```python
from build123d import *

# Parameters (mm, degrees)
BOSS_EXTRUDE1_DEPTH            = 17
BOSS_EXTRUDE2_START            = 17
SKETCH1_3_W                    = 18
SKETCH1_3_H                    = 7.7
BOSS_EXTRUDE2_DEPTH            = 8
SKETCH9_W                      = 65
SKETCH9_H                      = 70
CUT_EXTRUDE5_DEPTH             = 2
CBORE_FOR_M3_SHCS2_D           = 3.4
CBORE_FOR_M3_SHCS2_CBORE_D     = 6.5
CBORE_FOR_M3_SHCS2_CBORE_DEPTH = 3
SKETCH4_R                      = 1
CUT_EXTRUDE3_DEPTH             = 0.7
CUT_EXTRUDE4_DEPTH             = 0.5
CUT_EXTRUDE4_DEPTH_BACK        = 1
SKETCH6_W                      = 23.342383579
SKETCH6_H                      = 4
CBORE_FOR_M2_SHCS1_D           = 2.4
CBORE_FOR_M2_SHCS1_CBORE_D     = 4.4
CBORE_FOR_M2_SHCS1_CBORE_DEPTH = 2
FILLET1_R                      = 4


with BuildPart() as part:
    # Sketch1 → Boss-Extrude1 (new body)
    with BuildSketch(Plane(origin=(0, 0, 0), x_dir=(1, 0, 0), z_dir=(0, 1, 0))):
        Polygon((32.5, 0.5), (32.5, 70), (15, 90), (-15, 90), (-32.5, 70), (-32.5, -7.7), (-14.5, -7.7), (-14.5, 0), (14.1, 0), (14.1, 0.5), align=None)
    extrude(amount=BOSS_EXTRUDE1_DEPTH)

    # Sketch1<3> → Boss-Extrude2 (add)
    with BuildSketch(Plane(origin=(0, 0, 0), x_dir=(1, 0, 0), z_dir=(0, 1, 0)).offset(BOSS_EXTRUDE2_START)):
        with Locations((-23.5, -3.85)):
            Rectangle(SKETCH1_3_W, SKETCH1_3_H)
    extrude(amount=BOSS_EXTRUDE2_DEPTH)

    # Sketch9 → Cut-Extrude5 (cut)
    with BuildSketch(Plane(origin=(0, 17, 0), x_dir=(1, 0, 0), z_dir=(0, 1, 0))):
        with Locations((0, 35)):
            Rectangle(SKETCH9_W, SKETCH9_H)
    extrude(amount=-CUT_EXTRUDE5_DEPTH, mode=Mode.SUBTRACT)

    # CBORE for M3 SHCS2 (through all)
    with Locations(Plane(origin=(0, 15, 0), x_dir=(1, 0, 0), z_dir=(0, 1, 0))):
        with Locations((-5.12, 20), (12.88, 20), (-5.12, 63.6), (12.88, 63.6), (12.88, 5), (12.88, 48.6)):
            CounterBoreHole(CBORE_FOR_M3_SHCS2_D / 2, CBORE_FOR_M3_SHCS2_CBORE_D / 2, CBORE_FOR_M3_SHCS2_CBORE_DEPTH)

    # Sketch4 → Cut-Extrude3 (cut)
    with BuildSketch(Plane(origin=(0, 0, 0), x_dir=(0, 0, -1), z_dir=(1, 0, 0))):
        with BuildLine():
            ThreePointArc((78.521450009, 2.853281834), (77.510842566, 2.872195508), (77, 2))
            Line((77, 2), (78, 2))
            Line((78, 2), (78.521450009, 2.853281834))
        make_face()
        with BuildLine():
            Line((78, 2), (77, 2))
            ThreePointArc((77, 2), (78, 1), (79, 2))
            ThreePointArc((79, 2), (78.872195508, 2.489157434), (78.521450009, 2.853281834))
            Line((78.521450009, 2.853281834), (78, 2))
        make_face()
        with BuildLine():
            Line((58.012399764, 2.853281834), (57.490949754, 2))
            Line((57.490949754, 2), (58.490949754, 2))
            ThreePointArc((58.490949754, 2), (58.363145263, 2.489157434), (58.012399764, 2.853281834))
        make_face()
        with BuildLine():
            Line((58.490949754, 2), (57.490949754, 2))
            Line((57.490949754, 2), (58.012399764, 2.853281834))
            ThreePointArc((58.012399764, 2.853281834), (56.618754246, 1.510842566), (58.490949754, 2))
        make_face()
        with Locations((57.490949754, 2)):
            Circle(SKETCH4_R)
        with Locations((78, 2)):
            Circle(SKETCH4_R)
        Polygon((57.490949754, 2), (78, 2), (89, 20), (68.490949754, 20), align=None)
    extrude(amount=-CUT_EXTRUDE3_DEPTH, mode=Mode.SUBTRACT)

    # Sketch6 → Cut-Extrude4 (cut, two sides: drawn at the far end of the back side and taken through both)
    with BuildSketch(Plane.ZY.offset(-CUT_EXTRUDE4_DEPTH_BACK)):
        with Locations((-77.828808211, 15)):
            Rectangle(SKETCH6_W, SKETCH6_H)
    extrude(amount=CUT_EXTRUDE4_DEPTH + CUT_EXTRUDE4_DEPTH_BACK, mode=Mode.SUBTRACT)

    # CBORE for M2 SHCS1 (through all)
    with Locations(Plane(origin=(0, 0, 0), x_dir=(-1, 0, 0), z_dir=(0, 0, -1))):
        with Locations((22.5, 20.24)):
            CounterBoreHole(CBORE_FOR_M2_SHCS1_D / 2, CBORE_FOR_M2_SHCS1_CBORE_D / 2, CBORE_FOR_M2_SHCS1_CBORE_DEPTH)

    # Fillet1
    fillet1_edges = [part.edges().sort_by_distance(p)[0] for p in [
        (-32.5, 25, 3.85),
        (-14.5, 25, 3.85),
    ]]
    fillet(fillet1_edges, radius=FILLET1_R)


solid = part.part
```
Model file for the job. Use its own axes, mm. A direction names the side the tool comes from. Coordinates: 2 decimals unless noted, no trailing zeros. Loops run counter-clockwise (first coordinate to the right, second up) from the corner with the lowest first, then second, coordinate; pieces in that order, holes last. Notation, with made-up numbers: (54, 84.5) -> (69, 84.5) arc R27 ccw to (69, 101.5) -> close; hole circle Ø9 at (84, 6). An arc over 180 degrees is marked (long way). Answer as a JSON object with one key per item and string values.
Q1. Cut at D-D (y = 8.5). List the corners of the cut face in (x, z).
Report:
{"outline": "(-32.5, -70) -> (-15, -90) -> (15, -90) -> (32.5, -70) -> (32.5, -0.5) -> (14.1, -0.5) -> (14.1, 0) -> (-14.5, 0) -> (-14.5, 7.7) -> (-32.5, 7.7) -> close; hole circle Ø3.4 at (-5.12, -63.6); hole circle Ø3.4 at (-5.12, -20); hole (-0.7, -81.97) -> (0, -81.97) -> (0, -61.46) -> (-0.7, -61.46) -> close; hole circle Ø3.4 at (12.88, -63.6); hole circle Ø3.4 at (12.88, -48.6); hole circle Ø3.4 at (12.88, -20); hole circle Ø3.4 at (12.88, -5)"}
Q2. Cut at B-B (x = -5.12). List the corners of the cut face in (y, z).
Report:
{"outline": "(0, -90) -> (17, -90) -> (17, -70) -> (15, -70) -> (15, -66.85) -> (12, -66.85) -> (12, -65.3) -> (0, -65.3) -> close; (0, -61.9) -> (12, -61.9) -> (12, -60.35) -> (15, -60.35) -> (15, -23.25) -> (12, -23.25) -> (12, -21.7) -> (0, -21.7) -> close; (0, -18.3) -> (12, -18.3) -> (12, -16.75) -> (15, -16.75) -> (15, 0) -> (0, 0) -> close"}
Q3. Probe probe 1 along Z at (x, y) = (12.88, 8); probe 2 along Z at (x, y) = (12.88, 14.3); probe 3 along X at (y, z) = (13.5, -18.5). List the from-to ranges inside material, lowest first.
Report:
{"probe 1": "z = -90 to -65.3, -61.9 to -50.3, -46.9 to -21.7, -18.3 to -6.7, -3.3 to 0", "probe 2": "z = -90 to -66.85, -60.35 to -51.85, -45.35 to -23.25, -16.75 to -8.25, -1.75 to 0", "probe 3": "x = -32.5 to -8, -2.24 to 10, 15.76 to 32.5"}
Q4. Cut at A-A (z = -48.6). List the corners of the cut face in (x, y), and give its area (3 significant figures).
Report:
{"outline": "(-32.5, 0) -> (11.18, 0) -> (11.18, 12) -> (9.63, 12) -> (9.63, 15) -> (-32.5, 15) -> close; (14.58, 0) -> (32.5, 0) -> (32.5, 15) -> (16.13, 15) -> (16.13, 12) -> (14.58, 12) -> close", "area": "915 mm2"}
Q5. Cut at C-C (z = -63.6). List the corners of the cut face in (x, y), and give its area (3 significant figures).
Report:
{"outline": "(-32.5, 0) -> (-6.82, 0) -> (-6.82, 12) -> (-8.37, 12) -> (-8.37, 15) -> (-32.5, 15) -> close; (-3.42, 0) -> (11.18, 0) -> (11.18, 12) -> (9.63, 12) -> (9.63, 15) -> (-1.87, 15) -> (-1.87, 12) -> (-3.42, 12) -> close; (14.58, 0) -> (32.5, 0) -> (32.5, 15) -> (16.13, 15) -> (16.13, 12) -> (14.58, 12) -> close; hole (-0.7, 2) -> (0, 2) -> (0, 12) -> (-0.7, 12) -> close", "area": "847 mm2"}
Q6. 3-axis set-ups, long thin cutter, end or side, ignore diameter. For faces 1 (the flat face through (1, 15, -78)), 2 (the flat face through (0, 15, -35)), 3 (the flat face through (17, 16, -70)): which of +Z, -Z, +X, -X, +Y, -Y reach the whole face in a straight line?
Report:
{"face 1": "+Y", "face 2": "+X, -X, +Y", "face 3": "+Z, +X, -X, +Y"}
Q7. Flat gauge pins, fed straight in: P1, Ø5, axis at x = 14.5, z = -21.5, coming from the +Y side; P2, Ø5.5, axis at x = 12.88, z = -48.6, coming from the +Y side; P3, Ø1.5, axis at x = -18.5, y = 17, coming from the -Z side. Where does each tip first touch, or does it go through?
Report:
{"P1": "stops at y = 15", "P2": "stops at y = 12", "P3": "stops at z = -86.86"}
Q8. Pull direction X, two halves, no side cores. Call faces 4 (the cylindrical face through (-31.359, 23.797, 3.796)), 5 (the flat face through (-24, 12, 7.7)), 6 (the flat face through (-14.5, 10, 4)), 7 (the flat face through (-24, 20, 2)): released by +X, released by -X, zero draft, split by the parting line, or undercut.
Report:
{"face 4": "released by -X", "face 5": "zero draft", "face 6": "released by +X", "face 7": "undercut"}
